Autodesk Inventor part; units mm, degrees
ref_plane "YZ Plane" through (0, 0, 0) normal (1, 0, 0) x (0, 1, 0)
ref_plane "XZ Plane" through (0, 0, 0) normal (0, 1, 0) x (-1, 0, 0)
ref_plane "XY Plane" through (0, 0, 0) normal (0, 0, 1) x (1, 0, 0)
sketch "Sketch1" plane through (0, 0, 0) normal (0, 0, 1) x (1, 0, 0)
  circle A0 centre (0, 0) radius 4
  circle A1 centre (0, 0) radius 11
  line L0 (-25.9378, -1.7681) -> (-27.6396, -2.8187)
  line L1 (-27.6396, -2.8187) -> (-14.9069, -23.4452)
  line L2 (-14.9069, -23.4452) -> (-13.205, -22.3947)
  line L3 (0, 0) -> (11.913, 7.3539) construction
  circle A2 centre (0, 0) radius 14
  line L4 (-24, -20) -> (24, -20)
  line L5 (24, -20) -> (24, -25)
  line L6 (24, -25) -> (-24, -25)
  line L7 (-24, -25) -> (-24, -20)
  arc A3 (-14, -20) -> (-10.7276, -8.9954) centre (-16, -13.4164) ccw
  line L8 (-14, 0) -> (-14, -25) construction
  line L9 (0, 0) -> (-14, 0) construction
  line L10 (0, 0) -> (14, 0) construction
  line L11 (14, 0) -> (14, -25) construction
  arc A4 (10.7276, -8.9954) -> (14, -20) centre (16, -13.4164) ccw
  dimension "d0" = 8
  dimension "d1" = 22
  dimension "d19" = 3
  dimension "d20" = 25
  dimension "d21" = 5
  dimension "d22" = 2
  dimension "d23" = 2
  dimension "d24" = 10
  dimension "d25" = 10
extrude "Extrusion1" add sketch "Sketch1" along normal blind 7 contours A2 | A2 A4 L4 A3 | L4 L5 L6 L7
sketch "Sketch5" plane through (-24, -20, 0) normal (0, 1, 0) x (1, 0, 0)
  circle A0 centre (3, -3.5) radius 2
  circle A1 centre (45, -3.5) radius 2
  line L0 (3, -3.5) -> (45, -3.5) construction
  line L1 (0, 0) -> (0, -7)
  line L2 (48, 0) -> (48, -7)
  line L3 (10, 0) -> (0, 0)
  circle A2 centre (3, -3.5) radius 4.6098
  line L4 (0, 0) -> (48, 0)
  circle A3 centre (45, -3.5) radius 4.6098
  point P0 (24, 0)
  dimension "d26" = 4
  dimension "d27" = 4
  dimension "d28" = 3
  dimension "d29" = 3
  dimension "d30" = 3.5
extrude "Extrusion6" cut sketch "Sketch5" against normal up to surface (5 mm away) contours A0 | A1
extrude "Extrusion7" add sketch "Sketch5" against normal up to surface (5 mm away) contours L1 A2 | A3 L2
equation "\"d0\" = DIR"
equation "\"d1\" = DER"
equation "\"DER\" = 22"
equation "\"HR\" = 7"
equation "\"DIR\" = 8"
equation "\"DEM\" = 4"
equation "\"Dmarc\" = 17.5"
equation "\"Bsm\" = 22.5"
equation "\"Hsm\" = 12"
equation "\"Lsm\" = 21"
equation "\"Dsc\" = 5"
equation "\"RC\" = 6"
equation "\"PB\" = 25"
equation "\"TB\" = 3"
equation "\"HSE\" = 25"
equation "\"LMaSP\" = 46.5"
properties part number "SoportePolea"
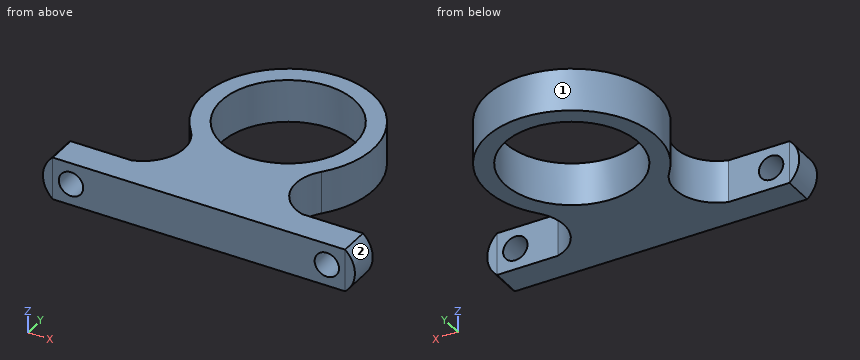
Source: CAD feature listing. Evaluate the final solid. Frame: model axes, mm. Face numbers are marked on the shaded views. Round coordinates to 2 decimals unless told otherwise and drop trailing zeros. Loops run counter-clockwise (first coordinate to the right, second up) from the corner with the lowest first, then second, coordinate; pieces in that order, holes last.
Q1. Section C-C, the plane y = 0. Return loops of the section in (x, z).
Q2. Ray query, line 1 (Z direction, x = -21, y = -21.45); line 2 (Y direction, x = -22, z = 1.25); line 3 (X direction, y = -22, z = 3). Return the intervals inside material, ascending.
Q3. Section B-B, the plane z = 3.5. Return loops of the section in (x, y), plus the area to 3 significant figures.
Q4. Mould query, pull axis Y, two halves, no side actions, for the marked faces 1 and 2. Classes: pulls with the +Y half, pulls with the -Y half, needs draft (parallel to the pull), parting line crosses it, or undercut.
Q5. Section A-A, the plane x = 21. Return loops of the section in (y, z).
Q6. First-contact query: P1, Ø0.8, axis at x = 25, z = 2, coming from the +Y side; P2, Ø4, axis at y = -19, z = 1.5, coming from the -X side. Flat tips, straight axial feed; report the tip coordinate or a pass-through.
Solutions:
1. outline: (-14, 0) - (-11, 0) - (-11, 7) - (-14, 7) - close; (11, 0) - (14, 0) - (14, 7) - (11, 7) - close
2. line 1: z = 0 to 1.5, 5.5 to 7
2. line 2: y = -25 to -20
2. line 3: x = -25.58 to -22.94, -19.06 to 19.06, 22.94 to 25.58
3. outline: (-25.61, -25) - (-23, -25) - (-23, -20) - (-25.61, -20) - close; (-19, -25) - (19, -25) - (19, -20) - (14, -20) arc R6.88 cw to (10.73, -9) arc R14 ccw (long way) to (-10.73, -9) arc R6.88 cw to (-14, -20) - (-19, -20) - close; (23, -25) - (25.61, -25) - (25.61, -20) - (23, -20) - close; hole circle Ø22 at (0, 0)
3. area: 599 mm2
4. face 1: undercut
4. face 2: needs draft
5. outline: (-25, 0) - (-20, 0) - (-20, 1.5) - (-25, 1.5) - close; (-25, 5.5) - (-20, 5.5) - (-20, 7) - (-25, 7) - close
6. P1: stops at y = -20
6. P2: stops at x = -25.6
